Here's how the part is built. I have some questions about the finished solid (model axes, mm). A direction names the side the tool comes from. Round coordinates to 2 decimals unless told otherwise and drop trailing zeros. Write each loop counter-clockwise with the first axis right and the second up, starting at its lowest first coordinate (ties: lowest second). Pieces come first, ordered by that corner, then holes. Notation, with made-up numbers: (81.25, 74) - (119.25, 74) arc R20 cw to (119.25, 98) - close; hole circle Ø6 at (47.5, -3.5). An arc over 180 degrees is marked (long way). Return JSON: item names as keys, results as strings. Group by question number.
```python
from build123d import *

# Parameters (mm, degrees)
SKETCH121_W      = 33
SKETCH121_H      = 33
EXTRUDE110_DEPTH = 4
SKETCH116_W      = 4
SKETCH116_H      = 36
SKETCH116_W_2    = 40
SKETCH116_H_2    = 4
SKETCH116_W_3    = 14
EXTRUDE105_DEPTH = 16.5
EXTRUDE104_DEPTH = 68.2


with BuildPart() as extrude110:
    # Sketch121 → Extrude110 (new body)
    with BuildSketch(Plane(origin=(0, 0, -13), x_dir=(1, 0, 0), z_dir=(0, 0, -1))):
        with Locations((32, -51)):
            Rectangle(SKETCH121_W, SKETCH121_H)
    extrude(amount=EXTRUDE110_DEPTH)


with BuildPart() as compound027:
    # Sketch116 → Extrude105 (new body)
    with BuildSketch(Plane.XY.offset(3)):
        with Locations((-1, 51)):
            Rectangle(SKETCH116_W, SKETCH116_H)
        with Locations((26, 80)):
            Rectangle(SKETCH116_W_2, SKETCH116_H_2)
        with Locations((13, 22)):
            Rectangle(SKETCH116_W_3, SKETCH116_H_2)
    extrude(amount=-EXTRUDE105_DEPTH)

    # Compound027: union Extrude110
    add(extrude110.part)


with BuildPart() as cut018:
    # Sketch115 → Extrude104 (new body)
    with BuildSketch(Plane.YZ.offset(-2.2)):
        Polygon((20.8, 1.5), (22.8, 1.5), (22.8, -13.5), (79.2, -13.5), (79.2, 1.5), (81.2, 1.5), (81.2, -15.5), (20.8, -15.5), align=None)
    extrude(amount=EXTRUDE104_DEPTH)

    # Cut018: cut Compound027
    add(compound027.part, mode=Mode.SUBTRACT)


solid = cut018.part
```
1) I need wall thicknesses on line 1 along Y through (x, z) = (51, -1.5); line 2 along X through (y, z) = (56, -14.5); line 3 along Z through (x, y) = (19, 30.5). Which ranges of each line are inside material? Lowest first, please.
2) Will these pins go through, and if not, where does the flat tip stop? pin 1 Ø8 at (y, z) = (66.5, -11.5) entering from -X; pin 2 Ø1.5 at (x, z) = (23, -3) entering from +Y; pin 3 Ø18 at (x, y) = (47.5, 62) entering from +Z.
3) If we mould it in two halves opening along Y, with no side actions, what happens to faces 6 (the flat face through (39, 20.8, -7)), 7 (the flat face through (31, 71, -13.5)), 8 (the flat face through (-2.2, 51, -15))? For each: released by +Y, released by -Y, zero draft, split by the parting line, or undercut.
4) Imagine slicing it at A-A (x = 41). Please give me the cut outline in (y, z).
5) Imagine slicing it at C-C (z = -2.75). Please give me the cut outline in (x, y), plus the area to 3 significant figures.
6) For faces 1 (the flat face through (48.5, 51, -14)), 2 (the flat face through (56, 79.2, -6)), 3 (the flat face through (6, 22, -6)), 4 (the flat face through (2, 80, 1.5)), 5 (the flat face through (46, 80, -6)), which set-ups out of +Z, -Z, +X, -X, +Y, -Y let a thin tool reach every point of the face, with its end or its side?
7) Imagine slicing it at B-B (y = 52.5). Please give me the cut outline in (x, z), plus the area to 3 significant figures.
8) Imagine slicing it at D-D (x = 60.5). Please give me the cut outline in (y, z).
Results found:
{
 "1": {"line 1": "y = 20.8 to 22.8, 79.2 to 81.2", "line 2": "x = -2.2 to 15.5, 48.5 to 66", "line 3": "z = -15.5 to -13.5"},
 "2": {"pin 1": "stops at x = -2.2", "pin 2": "stops at y = 22.8", "pin 3": "stops at z = -13.5"},
 "3": {"face 6": "released by -Y", "face 7": "undercut", "face 8": "zero draft"},
 "4": {"outline": "(20.8, -15.5) - (34.5, -15.5) - (34.5, -13.5) - (22.8, -13.5) - (22.8, 1.5) - (20.8, 1.5) - close; (67.5, -15.5) - (81.2, -15.5) - (81.2, -13.5) - (67.5, -13.5) - close"},
 "5": {"outline": "(-2.2, 20.8) - (6, 20.8) - (6, 22.8) - (-2.2, 22.8) - close; (-2.2, 79.2) - (6, 79.2) - (6, 81.2) - (-2.2, 81.2) - close; (20, 20.8) - (66, 20.8) - (66, 22.8) - (20, 22.8) - close; (46, 79.2) - (66, 79.2) - (66, 81.2) - (46, 81.2) - close", "area": "165 mm²"},
 "6": {"face 1": "+Z, -Z", "face 2": "+Z, +X, -X", "face 3": "+Z, +Y, -Y", "face 4": "+Z, +X, -X, +Y, -Y", "face 5": "+Z, +Y"},
 "7": {"outline": "(-2.2, -15.5) - (15.5, -15.5) - (15.5, -13.5) - (-2.2, -13.5) - close; (48.5, -15.5) - (66, -15.5) - (66, -13.5) - (48.5, -13.5) - close", "area": "70.4 mm²"},
 "8": {"outline": "(20.8, -15.5) - (81.2, -15.5) - (81.2, 1.5) - (79.2, 1.5) - (79.2, -13.5) - (22.8, -13.5) - (22.8, 1.5) - (20.8, 1.5) - close"}
}
